Source: CAD feature listing. Evaluate the final solid. Frame: model axes, mm. A direction names the side the tool comes from. Give positions to 0.01 mm unless a question says otherwise; leave off trailing zeros. Loops run counter-clockwise (first coordinate to the right, second up) from the corner with the lowest first, then second, coordinate; pieces in that order, holes last.
from build123d import *

# Parameters (mm, degrees)
SKETCH1_R           = 2.54
BOSS_EXTRUDE1_DEPTH = 5.08
SKETCH2_R           = 1.12
CUT_EXTRUDE1_DEPTH  = 3
SKETCH3_R           = 0.435
BOSS_EXTRUDE2_DEPTH = 2.5
FILLET1_R           = 0.1
FILLET2_R           = 0.1


with BuildPart() as part:
    # Sketch1 → Boss-Extrude1 (new body)
    with BuildSketch(Plane.XY):
        Circle(SKETCH1_R)
    extrude(amount=BOSS_EXTRUDE1_DEPTH)

    # Sketch2 → Cut-Extrude1 (cut)
    with BuildSketch(Plane.XY.offset(5.08)):
        Circle(SKETCH2_R)
    extrude(amount=-CUT_EXTRUDE1_DEPTH, mode=Mode.SUBTRACT)

    # Sketch3 → Boss-Extrude2 (add)
    with BuildSketch(Plane(origin=(0, 0, 0), x_dir=(-1, 0, 0), z_dir=(0, 0, -1))):
        Circle(SKETCH3_R)
    extrude(amount=BOSS_EXTRUDE2_DEPTH)

    # Fillet1
    fillet1_edges = [part.edges().sort_by_distance(p)[0] for p in [
        (0.435, 0, 0),
    ]]
    fillet(fillet1_edges, radius=FILLET1_R)

    # Fillet2
    fillet2_edges = [part.edges().sort_by_distance(p)[0] for p in [
        (0.435, 0, -2.5),
    ]]
    fillet(fillet2_edges, radius=FILLET2_R)


solid = part.part
1) Ray query, probe 1 along Y at (x, z) = (0, 4); probe 2 along Z at (x, y) = (0.15, -0.95); probe 3 along Z at (x, y) = (-0.6, -1.85). Return the intervals inside material, ascending.
Checks:
probe 1: y = -2.54 to -1.12, 1.12 to 2.54
probe 2: z = 0 to 2.08
probe 3: z = 0 to 5.08
2) Cut plane C-C (z = 4.25). Return loops of the section in (x, y), and give its area (3 significant figures).
Checks:
outline: circle Ø5.08 at (0, 0); hole circle Ø2.24 at (0, 0)
area: 16.3 mm2
3) Contact query for flat-ended pins moving along their axis: P1, Ø1, axis at y = 2, z = 2.5, coming from the -X side; P2, Ø1.5, axis at x = 1.5, z = 2, coming from the +Y side; P3, Ø1.5, axis at x = -1, z = 2.5, coming from the +Y side. Output: stop coordinate, or through.
Checks:
P1: stops at x = -2.05
P2: stops at y = 2.43
P3: stops at y = 2.53
4) Pull-direction query (Y, two-part tool) for faces 1 (the flat face through (0, 0, 2.08)), 2 (the cylindrical face through (-0.89, -0.68, 3.6)), 3 (the flat face through (0, 1, 0)), 4 (the cylindrical face through (-0.33, 2.52, 2.5)); classes: released by +Y, released by -Y, zero draft, split by the parting line, or undercut.
Checks:
face 1: undercut
face 2: undercut
face 3: zero draft
face 4: split by the parting line
5) Reachability of faces 5 (the cylindrical face through (0.094, -0.425, -1.234)), 6 (the flat face through (1, -1, 5.08)) from +Z, -Z, +X, -X, +Y, -Y: full face, straight path, thin tool, end or side. Return the list, or none.
Checks:
face 5: -Z
face 6: +Z, +X, -X, +Y, -Y
6) Cut plane D-D (z = -0.5). Return loops of the section in (x, y) (3 decimals).
Checks:
outline: circle Ø0.87 at (0, 0)
7) Cut plane A-A (y = 0). Return loops of the section in (x, z) (3 decimals), and give its area (3 significant figures).
Checks:
outline: (-2.54, 0) - (-0.535, 0) arc R0.1 cw to (-0.435, -0.1) - (-0.435, -2.4) arc R0.1 ccw to (-0.335, -2.5) - (0.335, -2.5) arc R0.1 ccw to (0.435, -2.4) - (0.435, -0.1) arc R0.1 cw to (0.535, 0) - (2.54, 0) - (2.54, 5.08) - (1.12, 5.08) - (1.12, 2.08) - (-1.12, 2.08) - (-1.12, 5.08) - (-2.54, 5.08) - close
area: 21.3 mm2
